Could you check a few things on this drawing? It's one solid part, dimensions in mm from its lowest x, y, z. Round coordinates to 2 decimals unless told otherwise and drop trailing zeros. Write each loop counter-clockwise with the first axis right and the second up, starting at its lowest first coordinate (ties: lowest second). Pieces come first, ordered by that corner, then holes. Notation, with made-up numbers: (65.25, 30.25) - (79.25, 30.25) arc R8 ccw to (79.25, 45.25) - close; hole circle Ø2 at (57, -37.75). An arc over 180 degrees is marked (long way). Use one line per item in the form item = value. Start each with the question number.
1. I want a section at C-C, the plane x = 8. List the corners of the cut face in (y, z) for me, plus the area to 3 significant figures.
2. I want a section at A-A, the plane y = 32. List the corners of the cut face in (x, z) for me.
3. If I drill on line 1 along Z through (x, y) = (8.5, 18.5); line 2 along X through (y, z) = (27.5, 34.5) (1 decimal); line 3 along X through (y, z) = (10, 47) (1 decimal), over which ranges is the centre line in solid material (lowest first)?
4. I want a section at B-B, the plane z = 38. List the corners of the cut face in (x, y) for me.
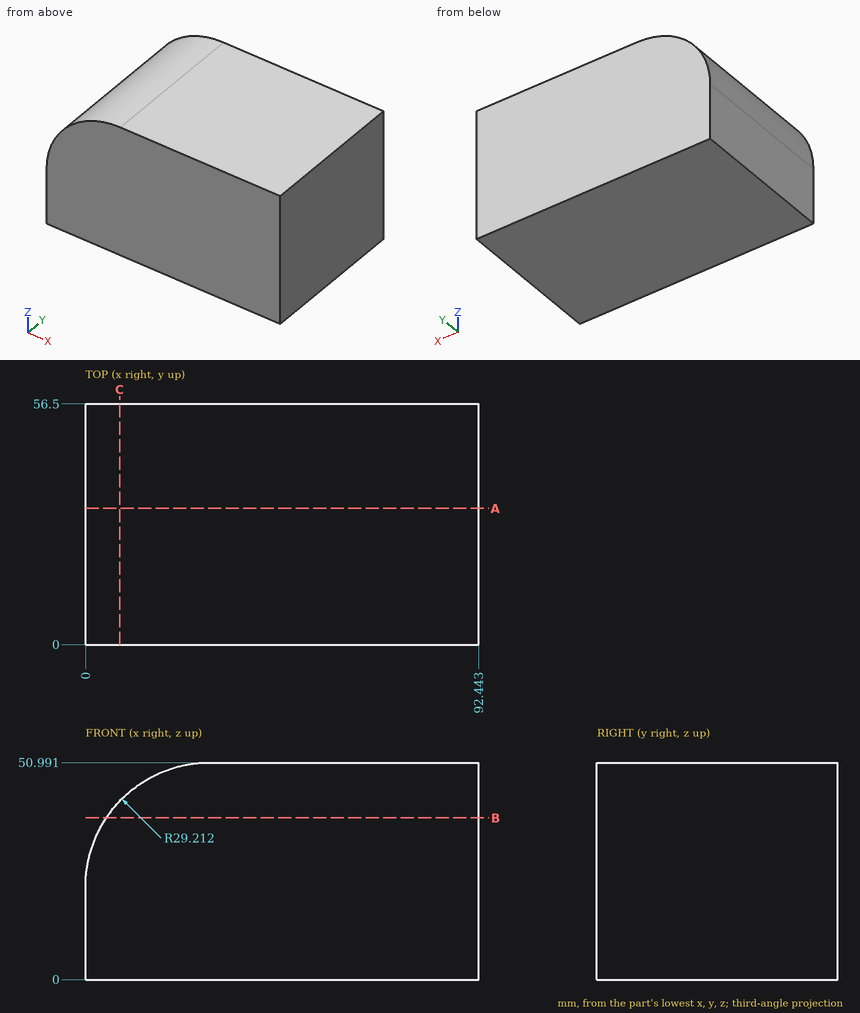
Model answer:
q1.outline = (0, 0) - (56.5, 0) - (56.5, 41.86) - (0, 41.86) - close
q1.area = 2,370 mm2
q2.outline = (0, 0) - (92.44, 0) - (92.44, 50.99) - (29.21, 50.99) arc R29.21 ccw to (0, 21.78) - close
q3.line_1 = 0 to 42.38
q3.line_2 = 2.9 to 92.4
q3.line_3 = 14.5 to 92.4
q4.outline = (4.92, 0) - (92.44, 0) - (92.44, 56.5) - (4.92, 56.5) - close
